from build123d import *

# Parameters (mm, degrees)
F0_W     = 165.1
F0_H     = 38.1
F1_DEPTH = 63.5
F2_W     = 156.972
F2_H     = 55.372
F3_DEPTH = 46.736
F4_W     = 165.1
F4_H     = 63.5
F5_DEPTH = 2.54


with BuildPart() as f1:
    # F0 (on Front) → F1 (new body)
    with BuildSketch(Plane.XZ):
        Rectangle(F0_W, F0_H)
    extrude(amount=F1_DEPTH)

    # F2 (on face) → F3 (cut)
    with BuildSketch(Plane.XY.offset(19.05)):
        with Locations((0, -31.75)):
            Rectangle(F2_W, F2_H)
    extrude(amount=-F3_DEPTH, mode=Mode.SUBTRACT)

    # F4 (on face) → F5 (join)
    with BuildSketch(Plane(origin=(0, 0, -19.05), x_dir=(1, 0, 0), z_dir=(0, 0, -1))):
        with Locations((0, 31.75)):
            Rectangle(F4_W, F4_H)
    extrude(amount=F5_DEPTH)


solid = f1.part
Source: CAD feature listing. Evaluate the final solid. Frame: model axes, mm. A direction names the side the tool comes from. Coordinates: 2 decimals unless noted, no trailing zeros. Order: outer loops, then holes, each group sorted by start corner. A loop starts at its lowest first (then second) coordinate and runs counter-clockwise, first axis right, second up.
Item 1: Cut plane B-B (y = -11). Return loops of the section in (x, z), plus the area to 3 significant figures.
Output values:
outline: (-82.55, -21.59) - (82.55, -21.59) - (82.55, 19.05) - (78.49, 19.05) - (78.49, -19.05) - (-78.49, -19.05) - (-78.49, 19.05) - (-82.55, 19.05) - close
area: 729 mm2
Item 2: Cut plane C-C (x = -8.5). Return loops of the section in (y, z).
Output values:
outline: (-63.5, -21.59) - (0, -21.59) - (0, 19.05) - (-4.06, 19.05) - (-4.06, -19.05) - (-59.44, -19.05) - (-59.44, 19.05) - (-63.5, 19.05) - close
Item 3: Pull-direction query (X, two-part tool) for faces 1 (the face through (-1, -59.436, 0)), 2 (the face through (-1, 0, -1)), 3 (the face through (78.486, -32, 0)), 4 (the face through (-82.55, -31, -1)); classes: pulls with the +X half, pulls with the -X half, needs draft (parallel to the pull), parting line crosses it, or undercut.
Output values:
face 1: undercut
face 2: needs draft
face 3: undercut
face 4: pulls with the -X half
Item 4: First-contact query: P1, Ø1, axis at x = -38.5, y = -19, coming from the +Z side. Flat tip, straight axial feed; report the tip coordinate or a pass-through.
Output values:
P1: stops at z = -19.05
Item 5: Set-up query: faces 5 (the face through (-7, -60, 19.05)), 6 (the face through (-1, -4.064, 0)). Return all of +Z, -Z, +X, -X, +Y, -Y with unobstructed straight access to the full face (end or side cutting, diameter ignored); none if empty.
Output values:
face 5: +Z, +X, -X, +Y, -Y
face 6: +Z
Item 6: Material intervals for line 1 (X direction, y = -31.5, z = -19); line 2 (Y direction, x = -2.5, z = 9.5); line 3 (Z direction, x = 76, y = -22.5), sorted ascending.
Output values:
line 1: x = -82.55 to -78.49, 78.49 to 82.55
line 2: y = -63.5 to -59.44, -4.06 to 0
line 3: z = -21.59 to -19.05
Item 7: Cut plane A-A (z = -17). Return loops of the section in (x, y), plus the area to 3 significant figures.
Output values:
outline: (-82.55, -63.5) - (82.55, -63.5) - (82.55, 0) - (-82.55, 0) - close; hole (-78.49, -59.44) - (78.49, -59.44) - (78.49, -4.06) - (-78.49, -4.06) - close
area: 1,790 mm2
